Autodesk Inventor part; units mm, degrees
ref_plane "YZ Plane" through (0, 0, 0) normal (1, 0, 0) x (0, 1, 0)
ref_plane "XZ Plane" through (0, 0, 0) normal (0, 1, 0) x (-1, 0, 0)
ref_plane "XY Plane" through (0, 0, 0) normal (0, 0, 1) x (1, 0, 0)
sketch "Sketch4" plane through (0, 0, 0) normal (0, 1, 0) x (-1, 0, 0)
  line L0 (0, 0) -> (-120, 0)
  line L1 (-120, 0) -> (-120, -20)
  line L2 (-120, -20) -> (0, -20)
  line L3 (0, -20) -> (0, 0)
  circle A0 centre (-15, -10) radius 2.5
  circle A1 centre (-40, -10) radius 2.5
  circle A2 centre (-65, -10) radius 2.5
  circle A3 centre (-110, -10) radius 2.5
  dimension "d6" = 120
  dimension "d7" = 20
  dimension "d11" = 5
  dimension "d12" = 5
  dimension "d13" = 5
  dimension "d14" = 5
  dimension "d15" = 10
  dimension "d16" = 15
  dimension "d17" = 25
  dimension "d18" = 25
extrude "Extrusion2" add sketch "Sketch4" along normal blind 2
fillet "Fillet2" radius 2 4 edges at (0, 1, -20) (0, 1, 0) (120, 1, 0) (120, 1, -20)
properties part number "Connector_H2"
Model file for the job. Use its own axes, mm. Coordinates: 2 decimals unless noted, no trailing zeros. Loops run counter-clockwise (first coordinate to the right, second up) from the corner with the lowest first, then second, coordinate; pieces in that order, holes last. Notation, with made-up numbers: (29, 41) -> (38, 41) arc R27 ccw to (38, 70) -> close; hole circle Ø9 at (41.5, 85). An arc over 180 degrees is marked (long way). Use one line per item in the form item = value. Start each with the question number.
(1) Cut at A-A on z = -10. Give the cut face in (x, y).
(2) Flat gauge pin, fed straight in: pin 1 (4 mm diameter, centred on x = 65, z = -10, fed in from -Y). Where does the tip first touch, or does it go through?
(3) Cut at C-C on x = 15. Give the cut face in (y, z), and give its area (3 significant figures).
(4) Cut at B-B on y = 0.6. Give the cut face in (x, z), and give its area (3 significant figures).
(5) Pull direction X, two halves, no side cores. Call faces 1 (the cylindrical face through (0.6, 1.01, -19.43)), 2 (the cylindrical face through (62.69, 0.99, -9.04)), 3 (the cylindrical face through (119.4, 1.01, -0.57)), 4 (the flat face through (61, 2, -10)): pulls with the +X half, pulls with the -X half, needs draft (parallel to the pull), parting line crosses it, or undercut.
(6) Probe probe 1 along Z at (x, y) = (15, 1.2); probe 2 along Z at (x, y) = (108.5, 0.4); probe 3 along X at (y, z) = (1.7, -9). List the from-to ranges inside material, lowest first. Write a range as from..to.
Values:
q1.outline = (0, 0) -> (12.5, 0) -> (12.5, 2) -> (0, 2) -> close; (17.5, 0) -> (37.5, 0) -> (37.5, 2) -> (17.5, 2) -> close; (42.5, 0) -> (62.5, 0) -> (62.5, 2) -> (42.5, 2) -> close; (67.5, 0) -> (107.5, 0) -> (107.5, 2) -> (67.5, 2) -> close; (112.5, 0) -> (120, 0) -> (120, 2) -> (112.5, 2) -> close
q2.pin_1 = through
q3.outline = (0, -20) -> (2, -20) -> (2, -12.5) -> (0, -12.5) -> close; (0, -7.5) -> (2, -7.5) -> (2, 0) -> (0, 0) -> close
q3.area = 30.0 mm2
q4.outline = (0, -18) arc R2 ccw to (2, -20) -> (118, -20) arc R2 ccw to (120, -18) -> (120, -2) arc R2 ccw to (118, 0) -> (2, 0) arc R2 ccw to (0, -2) -> close; hole circle Ø5 at (15, -10); hole circle Ø5 at (40, -10); hole circle Ø5 at (65, -10); hole circle Ø5 at (110, -10)
q4.area = 2,320 mm2
q5.face_1 = pulls with the -X half
q5.face_2 = undercut
q5.face_3 = pulls with the +X half
q5.face_4 = needs draft
q6.probe_1 = -20..-12.5, -7.5..0
q6.probe_2 = -20..-12, -8..0
q6.probe_3 = 0..12.71, 17.29..37.71, 42.29..62.71, 67.29..107.71, 112.29..120
